Design review of the part built by this model. Coordinates are the model's own, in mm. A direction names the side the tool comes from. Coordinates: 2 decimals unless noted, no trailing zeros. Order: outer loops, then holes, each group sorted by start corner. A loop starts at its lowest first (then second) coordinate and runs counter-clockwise, first axis right, second up. Notation, with made-up numbers: (69.5, -28) -> (85.5, -28) arc R16 cw to (85.5, -12) -> close; hole circle Ø6 at (-19.75, -11.5). An arc over 180 degrees is marked (long way). Use a Markdown table: item, result. Add a question column.
Q1. The part is to be moulded in two halves that separate along Z. For faces 6 (the face through (58.39, 7.31, 4.93)), 7 (the face through (23, 27, 18)), 8 (the face through (-9, 0, 16)), say which applies: pulls with the +Z half, pulls with the -Z half, needs draft (parallel to the pull), parting line crosses it, or undercut.
Q2. Add section D-D (y = 49.45). Count the separate pieces of the cut face and the enclosed holes in it, then the cut area to 3 significant figures.
Q3. Add section B-B (y = 0.45). State the section outline as (x, z) points, then the cut area to 3 significant figures.
Q4. Wall thickness on probe 1 along Y at (x, z) = (-23.45, 4); probe 2 along Y at (x, z) = (8.15, 4); probe 3 along X at (y, z) = (20, 15.5): over which ranges is each line inside the solid? List them lowest first.
Q5. Add section C-C (x = 8.15). State the section outline as (y, z) points.
Q6. Machinability: for faces 1 (the face through (54.5, 42, 9)), 2 (the face through (12, 11, 9)), 3 (the face through (-9, 49, 16)), 4 (the face through (-20.8, 49, 14)), 5 (the face through (58, 45, 10)), which of the approach directions +Z, -Z, +X, -X, +Y, -Y give a long, thin tool a straight path to every point of the face, cutting with its end or side? Answer none if there is none.
Q7. Insertion check: pin 1 (8 mm diameter, centred on x = 31.5, z = 7, fed in from -Y); pin 2 (9 mm diameter, centred on x = 23, z = 9, fed in from +Y); pin 3 (4 mm diameter, centred on y = 1, z = 4, fed in from -X); pin 4 (9 mm diameter, centred on y = 27.5, z = 12.5, fed in from -X). Each pin has a flat end and moves straight along its axis. Give the tip position at first contact, or say it passes through.
Q8. Add section A-A (y = 41). State the section outline as (x, z) points.
from build123d import *

# Parameters (mm, degrees)
SKETCH2_W                = 66.5
SKETCH2_H                = 55
SKETCH2_W_2              = 42.5
SKETCH2_H_2              = 20.5
BOSS_EXTRUDE1_DEPTH      = 18
SKETCH5_W                = 2
SKETCH5_H                = 6
BOSS_EXTRUDE2_DEPTH      = 26.8
BOSS_EXTRUDE3_REACH      = 89.768
SKETCH6_W                = 3
SKETCH6_H                = 6
SKETCH6_W_2              = 2
CUT_EXTRUDE3_REACH       = 90.155
SKETCH8_W                = 42
SKETCH8_H                = 4.25
SKETCH8_W_2              = 42.5
SKETCH12_W               = 3
SKETCH12_H               = 6
BOSS_EXTRUDE7_DEPTH      = 14
SKETCH14_W               = 4
SKETCH14_H               = 6
BOSS_EXTRUDE8_DEPTH      = 16.8
BOSS_EXTRUDE9_DEPTH      = 14
BOSS_EXTRUDE9_DEPTH_BACK = 1
SKETCH17_W               = 23.8
SKETCH17_H               = 6
SKETCH18_W               = 19.8
SKETCH18_H               = 14
CUT_EXTRUDE4_DEPTH       = 10
SKETCH20_W               = 5
SKETCH20_H               = 14
BOSS_EXTRUDE10_DEPTH     = 6
SKETCH22_W               = 38.8
SKETCH22_H               = 18
BOSS_EXTRUDE11_DEPTH     = 1
SKETCH23_W               = 26.8
SKETCH23_H               = 18
BOSS_EXTRUDE12_DEPTH     = 1
BOSS_EXTRUDE13_DEPTH     = 1
SKETCH25_W               = 12
SKETCH25_H               = 18
BOSS_EXTRUDE14_DEPTH     = 1
SKETCH27_W               = 38.8
SKETCH27_H               = 18
SKETCH27_W_2             = 19.8
SKETCH27_H_2             = 14
BOSS_EXTRUDE15_DEPTH     = 1
SKETCH28_W               = 12
SKETCH28_H               = 18
BOSS_EXTRUDE16_DEPTH     = 1
SKETCH32_W               = 18
SKETCH32_H               = 2.75
CUT_EXTRUDE8_DEPTH       = 26.8
SKETCH33_W               = 38.8
SKETCH33_H               = 18
SKETCH33_W_2             = 19.8
SKETCH33_H_2             = 14
BOSS_EXTRUDE17_DEPTH     = 2.75
SKETCH34_W               = 12
SKETCH34_H               = 18
BOSS_EXTRUDE18_DEPTH     = 2.75
SKETCH35_W               = 26.8
SKETCH35_H               = 18
BOSS_EXTRUDE19_DEPTH     = 2.3
SKETCH36_W               = 12
SKETCH36_H               = 18
SKETCH36_W_2             = 38.8
CUT_EXTRUDE9_DEPTH       = 2.75
SKETCH37_R               = 2.5
CUT_EXTRUDE10_DEPTH      = 6
SKETCH39_R               = 2.5
CUT_EXTRUDE12_DEPTH      = 10
SKETCH38_R               = 2.5
CUT_EXTRUDE11_DEPTH      = 6
SKETCH40_W               = 0.5
SKETCH40_H               = 4.25
CUT_EXTRUDE13_DEPTH      = 18
BOSS_EXTRUDE21_DEPTH     = 0.45
SKETCH44_R               = 5.25
BOSS_EXTRUDE22_DEPTH     = 12
SKETCH45_W               = 14
SKETCH45_H               = 8.45
BOSS_EXTRUDE23_DEPTH     = 2
CUT_EXTRUDE14_DEPTH      = 95.506891283
FILLET1_R                = 0.5


with BuildPart() as part:
    # Sketch2 → Boss-Extrude1 (new body)
    with BuildSketch(Plane.XY):
        with Locations((33.25, 27.5)):
            Rectangle(SKETCH2_W, SKETCH2_H)
        with Locations((33.25, 40.5)):
            Rectangle(SKETCH2_W_2, SKETCH2_H_2, mode=Mode.SUBTRACT)
        with Locations((33.25, 14.5)):
            Rectangle(SKETCH2_W_2, SKETCH2_H_2, mode=Mode.SUBTRACT)
    extrude(amount=BOSS_EXTRUDE1_DEPTH)

    # Sketch5 → Boss-Extrude2 (add)
    with BuildSketch(Plane.ZY):
        with Locations((1, 52)):
            Rectangle(SKETCH5_W, SKETCH5_H)
        with Locations((17, 52)):
            Rectangle(SKETCH5_W, SKETCH5_H)
        with Locations((1, 3)):
            Rectangle(SKETCH5_W, SKETCH5_H)
        with Locations((17, 3)):
            Rectangle(SKETCH5_W, SKETCH5_H)
    extrude(amount=BOSS_EXTRUDE2_DEPTH)

    # Sketch6 → Boss-Extrude3 (add, up to next)
    with BuildSketch(Plane.XY.offset(2), mode=Mode.PRIVATE) as boss_extrude3_sk1:
        with Locations((-25.3, 52)):
            Rectangle(SKETCH6_W, SKETCH6_H)
    boss_extrude3_tool1 = extrude(boss_extrude3_sk1.sketch, amount=BOSS_EXTRUDE3_REACH, mode=Mode.PRIVATE) - part.part
    # Sketch6 → Boss-Extrude3 (add, up to next)
    with BuildSketch(Plane.XY.offset(2), mode=Mode.PRIVATE) as boss_extrude3_sk2:
        with Locations((-25.8, 3)):
            Rectangle(SKETCH6_W_2, SKETCH6_H)
    boss_extrude3_tool2 = extrude(boss_extrude3_sk2.sketch, amount=BOSS_EXTRUDE3_REACH, mode=Mode.PRIVATE) - part.part
    add(boss_extrude3_tool1.solids().sort_by_distance((-25.3, 52, 2))[0])
    add(boss_extrude3_tool2.solids().sort_by_distance((-25.8, 3, 2))[0])

    # Sketch8 → Cut-Extrude3 (cut, up to next)
    with BuildSketch(Plane.XY.offset(18), mode=Mode.PRIVATE) as cut_extrude3_sk1:
        with Locations((33, 52.875)):
            Rectangle(SKETCH8_W, SKETCH8_H)
    cut_extrude3_tool1 = extrude(cut_extrude3_sk1.sketch, amount=-CUT_EXTRUDE3_REACH, mode=Mode.PRIVATE) & part.part
    # Sketch8 → Cut-Extrude3 (cut, up to next)
    with BuildSketch(Plane.XY.offset(18), mode=Mode.PRIVATE) as cut_extrude3_sk2:
        with Locations((33.25, 2.125)):
            Rectangle(SKETCH8_W_2, SKETCH8_H)
    cut_extrude3_tool2 = extrude(cut_extrude3_sk2.sketch, amount=-CUT_EXTRUDE3_REACH, mode=Mode.PRIVATE) & part.part
    add(cut_extrude3_tool1.solids().sort_by_distance((33, 52.875, 18))[0], mode=Mode.SUBTRACT)
    add(cut_extrude3_tool2.solids().sort_by_distance((33.25, 2.125, 18))[0], mode=Mode.SUBTRACT)

    # Sketch12 → Boss-Extrude7 (add)
    with BuildSketch(Plane.XY.offset(2)):
        with Locations((-6.5, 3)):
            Rectangle(SKETCH12_W, SKETCH12_H)
    extrude(amount=BOSS_EXTRUDE7_DEPTH)

    # Sketch14 → Boss-Extrude8 (add)
    with BuildSketch(Plane.ZY.offset(8)):
        with Locations((9, 3)):
            Rectangle(SKETCH14_W, SKETCH14_H)
    extrude(amount=BOSS_EXTRUDE8_DEPTH)

    # Sketch17 → Boss-Extrude9 (add, two sides: drawn at the far end of the back side and taken through both)
    with BuildSketch(Plane.XY.offset(2).offset(-BOSS_EXTRUDE9_DEPTH_BACK)):
        with Locations((-11.9, 52)):
            Rectangle(SKETCH17_W, SKETCH17_H)
    extrude(amount=BOSS_EXTRUDE9_DEPTH + BOSS_EXTRUDE9_DEPTH_BACK)

    # Sketch18 → Cut-Extrude4 (cut)
    with BuildSketch(Plane(origin=(0, 6, 0), x_dir=(1, 0, 0), z_dir=(0, 1, 0))):
        with Locations((-14.9, -9)):
            Rectangle(SKETCH18_W, SKETCH18_H)
    extrude(amount=-CUT_EXTRUDE4_DEPTH, mode=Mode.SUBTRACT)

    # Sketch20 → Boss-Extrude10 (add)
    with BuildSketch(Plane(origin=(0, 6, 0), x_dir=(1, 0, 0), z_dir=(0, 1, 0))):
        with Locations((-22.3, -9)):
            Rectangle(SKETCH20_W, SKETCH20_H)
    extrude(amount=-BOSS_EXTRUDE10_DEPTH)

    # Sketch22 → Boss-Extrude11 (add)
    with BuildSketch(Plane(origin=(0, 55, 0), x_dir=(1, 0, 0), z_dir=(0, 1, 0))):
        with Locations((-7.4, -9)):
            Rectangle(SKETCH22_W, SKETCH22_H)
    extrude(amount=BOSS_EXTRUDE11_DEPTH)

    # Sketch23 → Boss-Extrude12 (add)
    with BuildSketch(Plane.XZ.offset(-49)):
        with Locations((-13.4, 9)):
            Rectangle(SKETCH23_W, SKETCH23_H)
    extrude(amount=BOSS_EXTRUDE12_DEPTH)

    # Sketch24 → Boss-Extrude13 (add)
    with BuildSketch(Plane(origin=(0, 6, 0), x_dir=(1, 0, 0), z_dir=(0, 1, 0))):
        Polygon((0, 0), (-26.8, 0), (-26.8, -18), (0, -18), (0, -16), (-19.8, -16), (-19.8, -2), (0, -2), align=None)
    extrude(amount=BOSS_EXTRUDE13_DEPTH)

    # Sketch25 → Boss-Extrude14 (add)
    with BuildSketch(Plane(origin=(0, 55, 0), x_dir=(1, 0, 0), z_dir=(0, 1, 0))):
        with Locations((60.5, -9)):
            Rectangle(SKETCH25_W, SKETCH25_H)
    extrude(amount=BOSS_EXTRUDE14_DEPTH)

    # Sketch27 → Boss-Extrude15 (add)
    with BuildSketch(Plane.XZ):
        with Locations((-7.4, 9)):
            Rectangle(SKETCH27_W, SKETCH27_H)
        with Locations((-9.9, 9)):
            Rectangle(SKETCH27_W_2, SKETCH27_H_2, mode=Mode.SUBTRACT)
    extrude(amount=BOSS_EXTRUDE15_DEPTH)

    # Sketch28 → Boss-Extrude16 (add)
    with BuildSketch(Plane.XZ):
        with Locations((60.5, 9)):
            Rectangle(SKETCH28_W, SKETCH28_H)
    extrude(amount=BOSS_EXTRUDE16_DEPTH)

    # Sketch32 → Cut-Extrude8 (cut)
    with BuildSketch(Plane.ZY.offset(26.8)):
        with Locations((9, 5.625)):
            Rectangle(SKETCH32_W, SKETCH32_H)
    extrude(amount=-CUT_EXTRUDE8_DEPTH, mode=Mode.SUBTRACT)

    # Sketch33 → Boss-Extrude17 (add)
    with BuildSketch(Plane.XZ.offset(1)):
        with Locations((-7.4, 9)):
            Rectangle(SKETCH33_W, SKETCH33_H)
        with Locations((-9.9, 9)):
            Rectangle(SKETCH33_W_2, SKETCH33_H_2, mode=Mode.SUBTRACT)
    extrude(amount=BOSS_EXTRUDE17_DEPTH)

    # Sketch34 → Boss-Extrude18 (add)
    with BuildSketch(Plane.XZ.offset(1)):
        with Locations((60.5, 9)):
            Rectangle(SKETCH34_W, SKETCH34_H)
    extrude(amount=BOSS_EXTRUDE18_DEPTH)

    # Sketch35 → Boss-Extrude19 (add)
    with BuildSketch(Plane.XZ.offset(-48)):
        with Locations((-13.4, 9)):
            Rectangle(SKETCH35_W, SKETCH35_H)
    extrude(amount=BOSS_EXTRUDE19_DEPTH)

    # Sketch36 → Cut-Extrude9 (cut)
    with BuildSketch(Plane(origin=(0, 56, 0), x_dir=(1, 0, 0), z_dir=(0, 1, 0))):
        with Locations((60.5, -9)):
            Rectangle(SKETCH36_W, SKETCH36_H)
        with Locations((-7.4, -9)):
            Rectangle(SKETCH36_W_2, SKETCH36_H)
    extrude(amount=-CUT_EXTRUDE9_DEPTH, mode=Mode.SUBTRACT)

    # Sketch37 → Cut-Extrude10 (cut)
    with BuildSketch(Plane.ZY.offset(26.8)):
        with Locations((4, 49.45)):
            Circle(SKETCH37_R)
        with Locations((14, 49.45)):
            Circle(SKETCH37_R)
    extrude(amount=-CUT_EXTRUDE10_DEPTH, mode=Mode.SUBTRACT)

    # Sketch39 → Cut-Extrude12 (cut)
    with BuildSketch(Plane(origin=(0, 0, 0), x_dir=(-1, 0, 0), z_dir=(0, 0, -1))):
        with Locations((-8.15, 19.75)):
            Circle(SKETCH39_R)
        with Locations((-8.15, 9.75)):
            Circle(SKETCH39_R)
        with Locations((-57.85, 19.75)):
            Circle(SKETCH39_R)
        with Locations((-57.85, 9.75)):
            Circle(SKETCH39_R)
        with Locations(Location((-8.15, 45.25, 0), (0, 0, 180))):
            Circle(SKETCH39_R)
        with Locations(Location((-8.15, 35.25, 0), (0, 0, 180))):
            Circle(SKETCH39_R)
        with Locations(Location((-57.85, 45.25, 0), (0, 0, 180))):
            Circle(SKETCH39_R)
        with Locations(Location((-57.85, 35.25, 0), (0, 0, 180))):
            Circle(SKETCH39_R)
    extrude(amount=-CUT_EXTRUDE12_DEPTH, mode=Mode.SUBTRACT)

    # Sketch38 → Cut-Extrude11 (cut)
    with BuildSketch(Plane.ZY.offset(26.8)):
        with Locations((4, 0.45)):
            Circle(SKETCH38_R)
        with Locations((14, 0.45)):
            Circle(SKETCH38_R)
    extrude(amount=-CUT_EXTRUDE11_DEPTH, mode=Mode.SUBTRACT)

    # Sketch40 → Cut-Extrude13 (cut)
    with BuildSketch(Plane(origin=(0, 0, 0), x_dir=(-1, 0, 0), z_dir=(0, 0, -1))):
        with Locations((-54.25, 52.875)):
            Rectangle(SKETCH40_W, SKETCH40_H)
    extrude(amount=-CUT_EXTRUDE13_DEPTH, mode=Mode.SUBTRACT)

    # Sketch43 → Boss-Extrude21 (add)
    with BuildSketch(Plane(origin=(0, 4.25, 0), x_dir=(1, 0, 0), z_dir=(0, 1, 0))):
        Polygon((0, 0), (-26.8, 0), (-26.8, -18), (0, -18), (0, -16), (-19.8, -16), (-19.8, -2), (0, -2), align=None)
    extrude(amount=BOSS_EXTRUDE21_DEPTH)

    # Sketch44 → Boss-Extrude22 (add)
    with BuildSketch(Plane(origin=(66.5, 0, 0), x_dir=(0, 0, -1), z_dir=(1, 0, 0))):
        with Locations(Location((-9, 14.75, 0), (0, 0, 180))):
            Circle(SKETCH44_R)
    extrude(amount=BOSS_EXTRUDE22_DEPTH)

    # Sketch45 → Boss-Extrude23 (add)
    with BuildSketch(Plane(origin=(-19.8, 0, 0), x_dir=(0, 0, -1), z_dir=(1, 0, 0))):
        with Locations((-9, 0.475)):
            Rectangle(SKETCH45_W, SKETCH45_H)
    extrude(amount=BOSS_EXTRUDE23_DEPTH)

    # Sketch48 → Cut-Extrude14 (cut, through all)
    with BuildSketch(Plane(origin=(0, 45.7, 0), x_dir=(-1, 0, 0), z_dir=(0, -1, 0))):
        Polygon((8.9, -16), (1.4, -16), (8.9, -10.101152658), (16.399963049, -16), align=None)
        Polygon((1.398571429, -2), (8.9, -7.9), (16.401428571, -2), align=None)
        Polygon((0, -3.2), (7.374285714, -9), (0, -14.8), align=None)
        Polygon((17.8, -3.195910825), (10.420515192, -9), (17.8, -14.804089175), align=None)
    extrude(amount=-CUT_EXTRUDE14_DEPTH, mode=Mode.SUBTRACT)

    # Fillet1
    fillet1_edges = [part.edges().sort_by_distance(p)[0] for p in [
        (0, 49.475, 14.8),
        (0, 49.475, 3.2),
        (-7.374285714, 49.475, 9),
        (-17.8, 49.475, 14.804089175),
        (-10.420515192, 49.475, 9),
        (-17.8, 49.475, 3.195910825),
        (-8.9, 49.475, 10.101152658),
        (-16.399963049, 49.475, 16),
        (-1.4, 49.475, 16),
        (-16.401428571, 49.475, 2),
        (-8.9, 49.475, 7.9),
        (-1.398571429, 49.475, 2),
    ]]
    fillet(fillet1_edges, radius=FILLET1_R)


solid = part.part
Established:
| question | item | result |
|---|---|---|
| 1 | face 6 | needs draft |
| 1 | face 7 | pulls with the +Z half |
| 1 | face 8 | undercut |
| 2 | separate pieces | 2 |
| 2 | enclosed holes | 4 |
| 2 | area | 683 mm^2 |
| 3 | outline | (-26.8, 0) -> (12, 0) -> (12, 18) -> (-26.8, 18) -> (-26.8, 16.5) -> (-20.8, 16.5) -> (-20.8, 11.5) -> (-26.8, 11.5) -> (-26.8, 6.5) -> (-20.8, 6.5) -> (-20.8, 1.5) -> (-26.8, 1.5) -> close; (54.5, 0) -> (66.5, 0) -> (66.5, 18) -> (54.5, 18) -> close; hole (-17.8, 2) -> (0, 2) -> (0, 16) -> (-17.8, 16) -> close |
| 3 | area | 605 mm^2 |
| 4 | probe 1 | -3.75 to -2.05, 2.95 to 4.7, 45.7 to 46.95, 51.95 to 53.25 |
| 4 | probe 2 | -3.75 to 7.25, 12.25 to 17.25, 22.25 to 32.75, 37.75 to 42.75, 47.75 to 53.25 |
| 4 | probe 3 | 0 to 12, 54.5 to 66.5 |
| 5 | outline | (-3.75, 0) -> (7.25, 0) -> (7.25, 10) -> (12.25, 10) -> (12.25, 0) -> (17.25, 0) -> (17.25, 10) -> (22.25, 10) -> (22.25, 0) -> (32.75, 0) -> (32.75, 10) -> (37.75, 10) -> (37.75, 0) -> (42.75, 0) -> (42.75, 10) -> (47.75, 10) -> (47.75, 0) -> (53.25, 0) -> (53.25, 18) -> (-3.75, 18) -> close |
| 6 | face 1 | +Z, -Z, +Y |
| 6 | face 2 | +Z, -Z, -Y |
| 6 | face 3 | +Y, -Y |
| 6 | face 4 | -X |
| 6 | face 5 | -Z |
| 7 | pin 1 | y = 24.75 |
| 7 | pin 2 | y = 30.25 |
| 7 | pin 3 | x = -26.8 |
| 7 | pin 4 | x = 0 |
| 8 | outline | (0, 0) -> (12, 0) -> (12, 18) -> (0, 18) -> close; (54.5, 0) -> (66.5, 0) -> (66.5, 18) -> (54.5, 18) -> close |
